Input: dimensioned drawing with shaded views. Units: mm. Origin: part minimum x, y, z. Round coordinates to 2 decimals unless told otherwise and drop trailing zeros. Order: outer loops, then holes, each group sorted by start corner. A loop starts at its lowest first (then second) coordinate and runs counter-clockwise, first axis right, second up. Notation, with made-up numbers: (-10.5, 68) - (9.5, 68) arc R32 ccw to (9.5, 94) - close; hole circle Ø3 at (58.25, -13.75). An arc over 180 degrees is marked (long way). One line per item, written item: value. Start each with the question number.
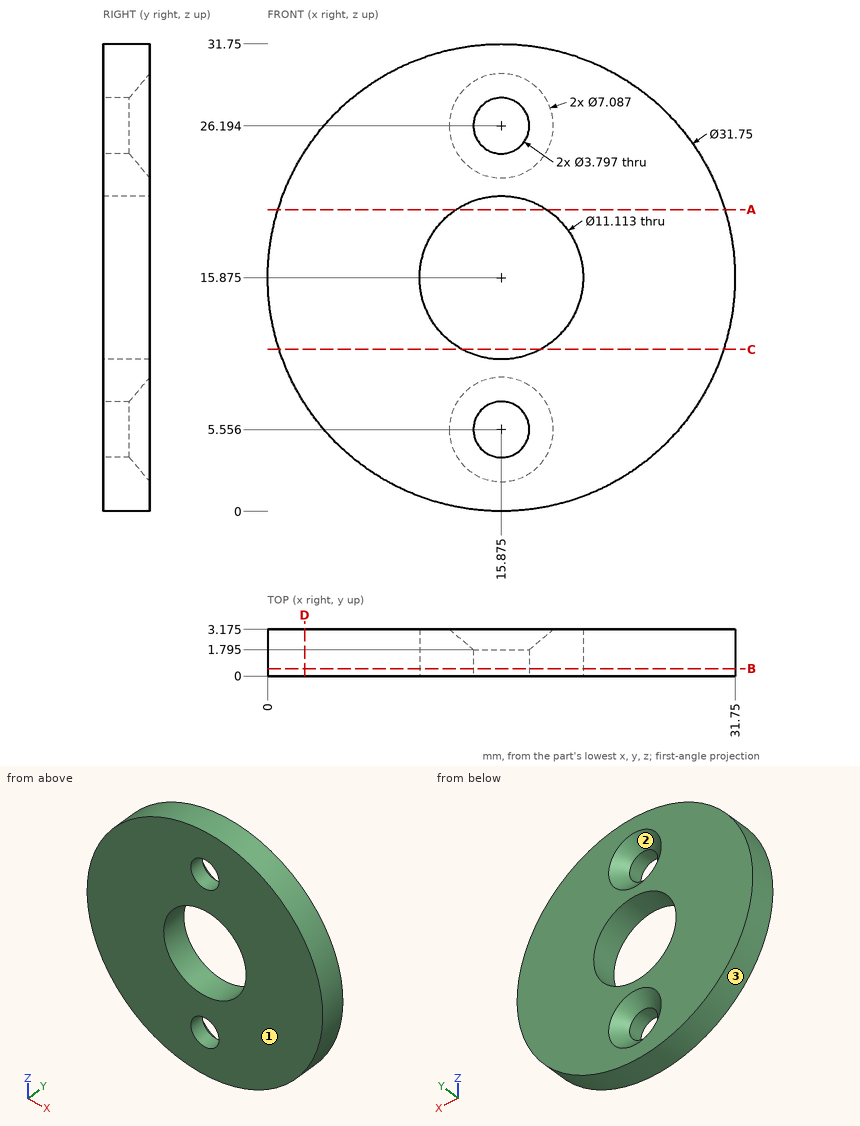
1. Pin query (flat end, axial travel): pin 1 (3.5 mm diameter, centred on x = 15.88, z = 26.19, fed in from -Y); pin 2 (1.5 mm diameter, centred on y = 0.5, z = 12.5, fed in from +X); pin 3 (4.5 mm diameter, centred on x = 15.88, z = 5.56, fed in from +Y) (1 decimal); pin 4 (1.5 mm diameter, centred on x = 12.5, y = 0.5, fed in from -Z). Return the tip coordinate at first contact, or that it passes through.
2. Pull-direction query (Z, two-part tool) for the marked faces 1, 2 and 3; classes: released by +Z, released by -Z, zero draft, split by the parting line, or undercut.
3. Section B-B (y = 0.5). State how many separate pieces and enclosed holes the cut face has, then the cut area to 3 significant figures.
4. Section C-C (z = 11). Return the cut outline in (x, y) (1 decimal).
5. Line query: line 1 (Z direction, x = 15, y = 0.5) (1 decimal); line 2 (Z direction, x = 15.5, y = 2) (1 decimal); line 3 (X direction, y = 0.35, z = 12.5) (1 decimal). Output: solid intervals per line, ascending. Write a range as from..to.
6. Section A-A (z = 20.5). Return the cut outline in (x, y) (1 decimal).
7. Section D-D (x = 2.5). Return the cut outline in (y, z) (1 decimal).
Solved:
1. pin 1: passes through
1. pin 2: stops at x = 31.53
1. pin 3: stops at y = 2.1
1. pin 4: stops at z = 0.22
2. face 1: zero draft
2. face 2: undercut
2. face 3: split by the parting line
3. separate pieces: 1
3. enclosed holes: 3
3. area: 672 mm²
4. outline: (0.8, 0) - (13.2, 0) - (13.2, 3.2) - (0.8, 3.2) - close; (18.5, 0) - (31, 0) - (31, 3.2) - (18.5, 3.2) - close
5. line 1: z = 0..3.9, 7.2..10.4, 21.4..24.5, 27.9..31.7
5. line 2: z = 0..3.4, 7.7..10.3, 21.4..24.1, 28.3..31.7
5. line 3: x = 0.4..11.5, 20.3..31.4
6. outline: (0.7, 0) - (12.8, 0) - (12.8, 3.2) - (0.7, 3.2) - close; (19, 0) - (31.1, 0) - (31.1, 3.2) - (19, 3.2) - close
7. outline: (0, 7.3) - (3.2, 7.3) - (3.2, 24.4) - (0, 24.4) - close
